from build123d import *

# Parameters (mm, degrees)
FILLET1_R                              = 5
M12_TAPPED_HOLE4_D                     = 10.2
M12_TAPPED_HOLE4_DEPTH                 = 29.25
M12_TAPPED_HOLE4_CSINK_D               = 12.05
M12_TAPPED_HOLE4_CSINK_ANGLE           = 90
M12_TAPPED_HOLE4_TIP                   = 3.064389157
M12_TAPPED_HOLE4_ON_FACE_2_D           = 10.2
M12_TAPPED_HOLE4_ON_FACE_2_DEPTH       = 29.25
M12_TAPPED_HOLE4_ON_FACE_2_CSINK_D     = 12.05
M12_TAPPED_HOLE4_ON_FACE_2_CSINK_ANGLE = 90
M12_TAPPED_HOLE4_ON_FACE_2_TIP         = 3.064389157


with BuildPart() as part:
    # Sketch1 → Revolve1 (revolve)
    with BuildSketch(Plane.XY, mode=Mode.PRIVATE) as revolve1_sk:
        Polygon((0, 0), (0, 20), (35, 20), (35, 50), (785, 50), (785, 20), (820, 20), (820, 0), align=None)
    revolve(revolve1_sk.sketch.rotate(Axis((820, 0, 0), (-1, 0, 0)), 90), axis=Axis((820, 0, 0), (-1, 0, 0)))

    # Fillet1
    fillet1_edges = [part.edges().sort_by_distance(p)[0] for p in [
        (785, 0, 20),
        (35, 0, 20),
    ]]
    fillet(fillet1_edges, radius=FILLET1_R)

    # M12 Tapped Hole4
    with Locations(Plane(origin=(0, 0, 0), x_dir=(0, 0, -1), z_dir=(-1, 0, 0))):
        with Locations((0, 0)):
            CounterSinkHole(M12_TAPPED_HOLE4_D / 2, M12_TAPPED_HOLE4_CSINK_D / 2, depth=M12_TAPPED_HOLE4_DEPTH, counter_sink_angle=M12_TAPPED_HOLE4_CSINK_ANGLE)
            with Locations((0, 0, -(M12_TAPPED_HOLE4_DEPTH + M12_TAPPED_HOLE4_TIP / 2))):  # 118° drill point
                Cone(0, M12_TAPPED_HOLE4_D / 2, M12_TAPPED_HOLE4_TIP, mode=Mode.SUBTRACT)

    # M12 Tapped Hole4 on face 2
    with Locations(Plane(origin=(820, 0, 0), x_dir=(0, 0, 1), z_dir=(1, 0, 0))):
        with Locations((0, 0)):
            CounterSinkHole(M12_TAPPED_HOLE4_ON_FACE_2_D / 2, M12_TAPPED_HOLE4_ON_FACE_2_CSINK_D / 2, depth=M12_TAPPED_HOLE4_ON_FACE_2_DEPTH, counter_sink_angle=M12_TAPPED_HOLE4_ON_FACE_2_CSINK_ANGLE)
            with Locations((0, 0, -(M12_TAPPED_HOLE4_ON_FACE_2_DEPTH + M12_TAPPED_HOLE4_ON_FACE_2_TIP / 2))):  # 118° drill point
                Cone(0, M12_TAPPED_HOLE4_ON_FACE_2_D / 2, M12_TAPPED_HOLE4_ON_FACE_2_TIP, mode=Mode.SUBTRACT)


solid = part.part
Here's how the part is built. I have some questions about the finished solid (model axes, mm). A direction names the side the tool comes from. Coordinates: 2 decimals unless noted, no trailing zeros. Loops run counter-clockwise (first coordinate to the right, second up) from the corner with the lowest first, then second, coordinate; pieces in that order, holes last.
1. For P1, Ø1.5, axis at x = 587, y = 36.5, coming from the +Z side; P2, Ø2, axis at y = -24, z = 7, coming from the -X side; P3, Ø4, axis at x = 736.5, z = 9, coming from the +Y side, each with a flat end and sliding along its axis, tell me the tip position at first contact or that it passes through.
2. If we mould it in two halves opening along Z, with no side actions, what happens to faces 4 (the cylindrical face through (415.25, -15.02, -47.69)), 5 (the flat face through (0, -5, 4))? For each: pulls with the +Z half, pulls with the -Z half, needs draft (parallel to the pull), parting line crosses it, or undercut.
3. For faces 1 (the flat face through (785, 10.4, 22.9)), 2 (the flat face through (35, 10.4, -22.9)), 3 (the flat face through (820, -5, -4)), which set-ups out of +Z, -Z, +X, -X, +Y, -Y let a thin tool reach every point of the face, with its end or its side?
4. I need wall thicknesses on L1, parallel to Y at x = 15, z = 0; L2, parallel to X at y = 6, z = -39; L3, parallel to Z at x = 527.5, y = -3. Which ranges of each line are inside material? Lowest first, please.
5. Imagine slicing it at A-A, the plane x = 397. Please give me the cut outline in (y, z), and give its area (3 significant figures).
6. Imagine slicing it at B-B, the plane z = -39. Please give me the cut outline in (x, y).
Taken from the geometry:
1. P1: stops at z = 34.96
1. P2: stops at x = 34.9
1. P3: stops at y = 49.51
2. face 4: parting line crosses it
2. face 5: needs draft
3. face 1: +X
3. face 2: -X
3. face 3: +Z, -Z, +X, +Y, -Y
4. L1: y = -20 to -5.1, 5.1 to 20
4. L2: x = 35 to 785
4. L3: z = -49.91 to 49.91
5. outline: circle Ø100 at (0, 0)
5. area: 7,850 mm2
6. outline: (35, -31.29) - (785, -31.29) - (785, 31.29) - (35, 31.29) - close
